from build123d import *

# Parameters (mm, degrees)
F0_W     = 285.75
F0_H     = 241.3
F1_DEPTH = 4.7625
F2_R     = 2.1
F3_DEPTH = 25.4
F4_W     = 25.4
F4_H     = 4.7625
F4_W_2   = 4.7625
F4_H_2   = 25.4
F5_DEPTH = 25.4


with BuildPart() as f1:
    # F0 (on Top) → F1 (new body)
    with BuildSketch(Plane.XY):
        Rectangle(F0_W, F0_H)
    extrude(amount=F1_DEPTH)

    # F2 (on face) → F3 (cut)
    with BuildSketch(Plane.XY.offset(4.7625)):
        with Locations((-89.737489, 77.047496)):
            Circle(F2_R)
        with Locations((-89.737489, 27.047495)):
            Circle(F2_R)
        with Locations((60.262516, 77.047496)):
            Circle(F2_R)
        with Locations((60.262516, 27.047495)):
            Circle(F2_R)
    extrude(amount=-F3_DEPTH, mode=Mode.SUBTRACT)

    # F4 (on face) → F5 (cut)
    with BuildSketch(Plane.XY.offset(4.7625)):
        with Locations((0, -118.26875)):
            Rectangle(F4_W, F4_H)
        with Locations((50.8, -118.26875)):
            Rectangle(F4_W, F4_H)
        with Locations((101.6, -118.26875)):
            Rectangle(F4_W, F4_H)
        with Locations((-50.8, -118.26875)):
            Rectangle(F4_W, F4_H)
        with Locations((-101.6, -118.26875)):
            Rectangle(F4_W, F4_H)
        with Locations((-101.6, 118.26875)):
            Rectangle(F4_W, F4_H)
        with Locations((-50.8, 118.26875)):
            Rectangle(F4_W, F4_H)
        with Locations((0, 118.26875)):
            Rectangle(F4_W, F4_H)
        with Locations((50.8, 118.26875)):
            Rectangle(F4_W, F4_H)
        with Locations((101.6, 118.26875)):
            Rectangle(F4_W, F4_H)
        with Locations((140.49375, 0)):
            Rectangle(F4_W_2, F4_H_2)
        with Locations((140.49375, 50.8)):
            Rectangle(F4_W_2, F4_H_2)
        with Locations((140.49375, 101.6)):
            Rectangle(F4_W_2, F4_H_2)
        with Locations((140.49375, -50.8)):
            Rectangle(F4_W_2, F4_H_2)
        with Locations((140.49375, -101.6)):
            Rectangle(F4_W_2, F4_H_2)
        with Locations((-140.49375, 101.6)):
            Rectangle(F4_W_2, F4_H_2)
        with Locations((-140.49375, 50.8)):
            Rectangle(F4_W_2, F4_H_2)
        with Locations((-140.49375, 0)):
            Rectangle(F4_W_2, F4_H_2)
        with Locations((-140.49375, -50.8)):
            Rectangle(F4_W_2, F4_H_2)
        with Locations((-140.49375, -101.6)):
            Rectangle(F4_W_2, F4_H_2)
    extrude(amount=-F5_DEPTH, mode=Mode.SUBTRACT)


solid = f1.part
For this review, take the finished solid that the model builds, in its own axes (mm). Give positions to 0.01 mm unless a question says otherwise; leave off trailing zeros. Order: outer loops, then holes, each group sorted by start corner. A loop starts at its lowest first (then second) coordinate and runs counter-clockwise, first axis right, second up. Notation, with made-up numbers: M -7,4.5 L 31,4.5 A33 cw 31,36.5 Z; hole C 50,-19.75 d4. An arc over 180 degrees is marked long. Answer in a Markdown table with one row per item. Add a question column.
(1) For pin 1 (1.4 mm diameter, centred on x = -104.5, z = 3, fed in from -Y); pin 2 (2.5 mm diameter, centred on x = 106, z = 2.5, fed in from +Y); pin 3 (2.5 mm diameter, centred on x = 60.26, y = 77.05, fed in from -Z), all flat-tipped, find the tip position at first contact; note any pin that passes through.
(2) Consider section A-A on x = -60. State the section outline as (y, z) points, and give its area (3 significant figures).
(3) Wall thickness on probe 1 along Y at (x, z) = (-7, 4.15); probe 2 along X at (y, z) = (76, 3.4) (3 decimals); probe 3 along X at (y, z) = (59.5, 1.55): over which ranges is each line inside the solid? List them lowest first. Write a range as [from, to].
(4) Consider section C-C on z = 1.55. Give the number of separate pieces and of enclosed holes in the cut face, and give its area (3 significant figures).
(5) Consider section B-B on y = 57. State the section outline as (x, z) points, and give its area (3 significant figures).
Evaluation:
| question | item | result |
|---|---|---|
| 1 | pin 1 | stops at y = -115.89 |
| 1 | pin 2 | stops at y = 115.89 |
| 1 | pin 3 | passes through |
| 2 | outline | M -115.89,0 L 115.89,0 L 115.89,4.76 L -115.89,4.76 Z |
| 2 | area | 1,100 mm^2 |
| 3 | probe 1 | y = [-115.89, 115.89] |
| 3 | probe 2 | x = [-142.875, -91.558], [-87.917, 58.442], [62.083, 142.875] |
| 3 | probe 3 | x = [-138.11, 138.11] |
| 4 | separate pieces | 1 |
| 4 | enclosed holes | 4 |
| 4 | area | 66,500 mm^2 |
| 5 | outline | M -138.11,0 L 138.11,0 L 138.11,4.76 L -138.11,4.76 Z |
| 5 | area | 1,320 mm^2 |
